Can you work these out from the model? Positions are in its coordinate system, mm. A direction names the side the tool comes from. Round coordinates to 2 decimals unless told otherwise and drop trailing zeros. Order: outer loops, then holes, each group sorted by start corner. A loop starts at its lowest first (then second) coordinate and runs counter-clockwise, first axis right, second up. Notation, with made-up numbers: M 1.25,-0.75 L 45.25,-0.75 A20 ccw 45.25,22.25 Z; hole C 2,7.25 d11. An arc over 180 degrees is marked long. Answer as a JSON object with one key per item and string values. Group by question number.
from build123d import *

# Parameters (mm, degrees)
PAD_DEPTH     = 90
SKETCH001_R   = 2.571292
SKETCH001_R_2 = 2.48503
POCKET_DEPTH  = 6


with BuildPart() as part:
    # Sketch → Pad (new body)
    with BuildSketch(Plane.YZ):
        Polygon((6, 0), (6, 30), (3, 30), (3, 23), (0, 25), (0, 5), (3, 7), (3, 0), align=None)
    extrude(amount=PAD_DEPTH)

    # Sketch001 → Pocket (cut)
    with BuildSketch(Plane(origin=(0, 0, 0), x_dir=(0, 0, -1), z_dir=(0, -1, 0))):
        with Locations((-15.088319, 45.037495)):
            Circle(SKETCH001_R)
        with Locations((-15.093687, 80.807022)):
            Circle(SKETCH001_R_2)
        with Locations((-15.089277, 10.18487)):
            Circle(SKETCH001_R_2)
    extrude(amount=-POCKET_DEPTH, mode=Mode.SUBTRACT)


solid = part.part
Item 1: Suppose I cut it at A-A, the plane x = 37.5. Write out the boundary of the cut face in (y, z), and give its area (3 significant figures).
Item 2: If we mould it in two halves opening along Z, with no side actions, what happens to faces 1 (the face through (7.98, 2.96, 13.94)), 2 (the face through (44, 6, 11)), 3 (the face through (44, 4, 0))? For each: +Z half, -Z half, draft (parallel to the pull), parting line (faces both ways), or undercut.
Item 3: I need wall thicknesses on line 1 (X direction, y = 0.65, z = 15); line 2 (X direction, y = 0.7, z = 17.25); line 3 (Y direction, x = 50, z = 5.5). Which ranges of each line are inside material? Lowest first, please.
Item 4: Suppose I cut it at C-C, the plane z = 27.25. Write out the boundary of the cut face in (x, y), and give its area (3 significant figures).
Item 5: Suppose I cut it at B-B, the plane y = 1.7. Write out the boundary of the cut face in (x, z), and give its area (3 significant figures).
Item 6: On a 3-axis mill with a long thin cutter (end or side, diameter ignored), from which of +Z, -Z, +X, -X, +Y, -Y can I reach the whole of each face in a straight line? I mean faces 4 (the face through (44, 0, 20)), 5 (the face through (44, 3, 27)). Say none if no direction works.
Item 7: I'm going to push flat-ended pins straight in: pin 1 Ø6 at (x, z) = (36, 3.5) entering from -Y; pin 2 Ø3.5 at (x, z) = (45.5, 27.5) entering from -Y. Where does each tip first touch, or does it pass through?
Computed:
{
 "1": {"outline": "M 0,5 L 3,7 L 3,0 L 6,0 L 6,30 L 3,30 L 3,23 L 0,25 Z", "area": "144 mm^2"},
 "2": {"face 1": "undercut", "face 2": "draft", "face 3": "-Z half"},
 "3": {"line 1": "x = 0 to 7.7, 12.67 to 42.47, 47.61 to 78.32, 83.29 to 90", "line 2": "x = 0 to 8.96, 11.41 to 43.65, 46.43 to 79.57, 82.04 to 90", "line 3": "y = 0 to 0.75, 3 to 6"},
 "4": {"outline": "M 0,3 L 90,3 L 90,6 L 0,6 Z", "area": "270 mm^2"},
 "5": {"outline": "M 0,6.13 L 90,6.13 L 90,23.87 L 0,23.87 Z; hole C 10.18,15.09 d4.97; hole C 45.04,15.09 d5.14; hole C 80.81,15.09 d4.97", "area": "1,540 mm^2"},
 "6": {"face 4": "+Z, -Z, +X, -X, -Y", "face 5": "+Z, +X, -X"},
 "7": {"pin 1": "stops at y = 0", "pin 2": "stops at y = 3"}
}
